from build123d import *

# Parameters (mm, degrees)
ESQUISSE1_R        = 1.75
ESQUISSE1_R_2      = 1.35
BOSS_EXTRU_1_DEPTH = 6
CHANFREIN1_SIZE    = 1.25
CONG_1_R           = 10


with BuildPart() as part:
    # Esquisse1 → Boss.-Extru.1 (new body)
    with BuildSketch(Plane.XY):
        with BuildLine():
            Line((0, 0), (49.546865916, 0))
            ThreePointArc((49.546865916, 0), (73.776718043, -15.184943457), (101.953496658, -10.312840336))
            ThreePointArc((101.953496658, -10.312840336), (107.75313821, -7.843303604), (114.000000849, -7))
            ThreePointArc((114.000000849, -7), (122.485281675, -3.485281074), (126, 5))
            ThreePointArc((126, 5), (124.535533906, 8.535533906), (121, 10))
            ThreePointArc((121, 10), (117.464466094, 8.535533906), (116, 5))
            ThreePointArc((116, 5), (115.414213863, 3.585786738), (114.000000849, 3))
            ThreePointArc((114.000000849, 3), (105.101532849, 1.798737416), (96.840117389, -1.719043012))
            ThreePointArc((96.840117389, -1.719043012), (73.408662827, -4.825876336), (55, 10))
            Line((55, 10), (0, 10))
            ThreePointArc((0, 10), (-5, 5), (0, 0))
        make_face()
        with Locations((0, 5)):
            Circle(ESQUISSE1_R, mode=Mode.SUBTRACT)
        with Locations((121, 5)):
            Circle(ESQUISSE1_R_2, mode=Mode.SUBTRACT)
    extrude(amount=BOSS_EXTRU_1_DEPTH)

    # Chanfrein1
    chanfrein1_edges = [part.edges().sort_by_distance(p)[0] for p in [
        (-1.75, 5, 0),
        (119.65, 5, 0),
    ]]
    chamfer(chanfrein1_edges, length=CHANFREIN1_SIZE)

    # Congé1
    cong_1_edges = [part.edges().sort_by_distance(p)[0] for p in [
        (49.546865916, 0, 3),
        (55, 10, 3),
    ]]
    fillet(cong_1_edges, radius=CONG_1_R)


solid = part.part
Work out the finished part from the listing and answer in its coordinate system (mm). A direction names the side the tool comes from. Round coordinates to 2 decimals unless told otherwise and drop trailing zeros. Write each loop counter-clockwise with the first axis right and the second up, starting at its lowest first coordinate (ties: lowest second). Pieces come first, ordered by that corner, then holes. Notation, with made-up numbers: (-30, -15) -> (25, -15) arc R21 cw to (25, 4) -> close; hole circle Ø1 at (-13, 9). An arc over 180 degrees is marked (long way). Answer as CSV lines item,"result". Start each with the question number.
(1) Find the intervals of material crossed by probe 1 along Y at (x, z) = (0, 3.65); probe 2 along X at (y, z) = (5.75, 5.65); probe 3 along X at (y, z) = (4, 2.3), in increasing order.
(2) This flat-tipped pin is pushed along its axis until it touches: pin 1 (1 mm diameter, centred on x = 18, z = 4.5, fed in from -Y). Where does it stop, or does it pass through?
(3) The part is cut by section B-B, the plane x = 40. Give the vertices of the cut face in (y, z).
(4) The mould has two halves that part along X. Classify faces 4 (the cylindrical face through (76.01, -5.43, 2.96)), 5 (the flat face through (60, 0, 6)), 6 (the cylindrical face through (75.451, -15.478, 2.958)): +X half, -X half, draft (parallel to the pull), parting line (faces both ways), or undercut.
(5) The part is cut by section A-A, the plane z = 3.15. Give the vertices of the cut face in (x, y), then the cut area to 3 significant figures.
(6) The part is cut by section C-C, the plane y = -8.75. Give the vertices of the cut face in (x, z).
(7) A tool of negligible diameter and unlimited length cuts with its end or side. For faces 1 (the flat face through (22, 0, 3)), 2 (the cylindrical face through (53.95, 8.98, 3.04)), 3 (the cylindrical face through (-0.38, 3.29, 3.59)), from which of +Z, -Z, +X, -X, +Y, -Y can it reach the whole face along a straight path? Write none if from no direction.
Output values:
1,probe 1,"y = 0 to 3.25, 6.75 to 10"
1,probe 2,"x = -4.94 to -1.58, 1.58 to 57.74, 116.06 to 119.88, 122.12 to 125.94"
1,probe 3,"x = -4.9 to -1.44, 1.44 to 59.2, 115.73 to 120.09, 121.91 to 125.96"
2,pin 1,"stops at y = 0"
3,outline,"(0, 0) -> (10, 0) -> (10, 6) -> (0, 6) -> close"
4,face 4,"undercut"
4,face 5,"draft"
4,face 6,"parting line"
5,outline,"(0, 0) -> (44.9, 0) arc R10 cw to (52.22, -3.19) arc R40 ccw to (101.95, -10.31) arc R23.56 cw to (114, -7) arc R12 ccw to (126, 5) arc R5 ccw to (116, 5) arc R2 cw to (114, 3) arc R33.56 ccw to (96.84, -1.72) arc R30 cw to (57.54, 6.02) arc R10 ccw to (49.55, 10) -> (0, 10) arc R5 ccw to start; hole circle Ø3.5 at (0, 5); hole circle Ø2.7 at (121, 5)"
5,area,"1,380 mm²"
6,outline,"(58.62, 0) -> (105.09, 0) -> (105.09, 6) -> (58.62, 6) -> close"
7,face 1,"+Z, -Z, -X, -Y"
7,face 2,"+Z, -Z, +Y"
7,face 3,"+Z, -Z"
